```python
from build123d import *

# Parameters (mm, degrees)
SKETCH20_W            = 96.52
SKETCH20_H            = 108.5559932
BOSS_EXTRUDE5_DEPTH   = 1.699999902
BOSS_EXTRUDE6_DEPTH   = 1.7
FILLET3_R             = 2.54
F_4_40_TAPPED_HOLE3_D = 2.2606
SKETCH28_W            = 11.938
SKETCH28_H            = 11.938
SKETCH28_W_2          = 5.08
SKETCH28_H_2          = 5.08
SKETCH28_W_3          = 51.308
SKETCH28_H_3          = 77.978
SKETCH28_R            = 1.27
CUT_EXTRUDE1_DEPTH    = 8.89


with BuildPart() as part:
    # Sketch20 → Boss-Extrude5 (new body)
    with BuildSketch(Plane(origin=(0, 0, 0), x_dir=(1, 0, 0), z_dir=(0, 1, 0))):
        with Locations((46.26, 74.0579966)):
            Rectangle(SKETCH20_W, SKETCH20_H)
    extrude(amount=-BOSS_EXTRUDE5_DEPTH)

    # Sketch20_3 → Boss-Extrude6 (add)
    with BuildSketch(Plane(origin=(0, 0, 0), x_dir=(1, 0, 0), z_dir=(0, 1, 0))):
        with BuildLine():
            Line((2.572, 21.812), (89.948, 21.812))
            ThreePointArc((89.948, 21.812), (90.691948776, 23.608051224), (92.488, 24.352))
            Line((92.488, 24.352), (92.488, 123.7639932))
            ThreePointArc((92.488, 123.7639932), (90.691948776, 124.507941976), (89.948, 126.3039932))
            Line((89.948, 126.3039932), (2.572, 126.3039932))
            ThreePointArc((2.572, 126.3039932), (1.828051224, 124.507941976), (0.032, 123.7639932))
            Line((0.032, 123.7639932), (0.032, 24.352))
            ThreePointArc((0.032, 24.352), (1.828051224, 23.608051224), (2.572, 21.812))
        make_face()
        with BuildLine():
            Line((3.624102448, 23.082), (88.895897552, 23.082))
            ThreePointArc((88.895897552, 23.082), (89.793923164, 24.506076836), (91.218, 25.404102448))
            Line((91.218, 25.404102448), (91.218, 122.711890752))
            ThreePointArc((91.218, 122.711890752), (89.793923164, 123.609916364), (88.895897552, 125.0339932))
            Line((88.895897552, 125.0339932), (3.624102448, 125.0339932))
            ThreePointArc((3.624102448, 125.0339932), (2.726076836, 123.609916364), (1.302, 122.711890752))
            Line((1.302, 122.711890752), (1.302, 25.404102448))
            ThreePointArc((1.302, 25.404102448), (2.726076836, 24.506076836), (3.624102448, 23.082))
        make_face(mode=Mode.SUBTRACT)
    extrude(amount=BOSS_EXTRUDE6_DEPTH)

    # Fillet3
    fillet3_edges = [part.edges().sort_by_distance(p)[0] for p in [
        (-2, -0.849999951, -128.3359932),
        (-2, -0.849999951, -19.78),
        (94.52, -0.849999951, -19.78),
        (94.52, -0.849999951, -128.3359932),
    ]]
    fillet(fillet3_edges, radius=FILLET3_R)

    # 4-40 Tapped Hole3 (through all)
    with Locations(Plane(origin=(0, 0, 0), x_dir=(1, 0, 0), z_dir=(0, 1, 0))):
        with Locations((0.032, 21.812), (92.488, 21.812), (92.488, 126.3039932), (0.032, 126.3039932)):
            Hole(F_4_40_TAPPED_HOLE3_D / 2)

    # Sketch28 → Cut-Extrude1 (cut)
    with BuildSketch(Plane.XZ.offset(1.699999902)):
        with Locations((11.843, -110.331)):
            Rectangle(SKETCH28_W, SKETCH28_H)
        with Locations((10.954, -77.692)):
            Rectangle(SKETCH28_W_2, SKETCH28_H_2)
        with Locations((55.658, -74.009)):
            Rectangle(SKETCH28_W_3, SKETCH28_H_3)
        with Locations((87.662, -118.078)):
            Circle(SKETCH28_R)
        with Locations((87.662, -29.94)):
            Circle(SKETCH28_R)
        with Locations((23.019, -118.078)):
            Circle(SKETCH28_R)
        with Locations((23.019, -29.94)):
            Circle(SKETCH28_R)
    extrude(amount=-CUT_EXTRUDE1_DEPTH, mode=Mode.SUBTRACT)


solid = part.part
```
Model file for the job. Use its own axes, mm. A direction names the side the tool comes from. Round coordinates to 2 decimals unless told otherwise and drop trailing zeros. Loops run counter-clockwise (first coordinate to the right, second up) from the corner with the lowest first, then second, coordinate; pieces in that order, holes last. Notation, with made-up numbers: M 75,47.25 L 118,47.25 A18 ccw 118,72.25 Z; hole C 49.5,87 d4. An arc over 180 degrees is marked long. Put each result on its own line as item: value. Start each with the question number.
Item 1: Cut at C-C (z = -29.94). List the corners of the cut face in (x, y).
Item 2: Cut at A-A (z = -114.5). List the corners of the cut face in (x, y), then the cut area to 3 significant figures.
Item 3: Drill centre lines: line 1 along X through (y, z) = (-0.85, -106); line 2 along X through (y, z) = (0.9, -94.5); line 3 along Z through (x, y) = (38.5, 0.85). Where is each one in solid material? Low to high.
Item 4: Drop flat-ended pins along their axis: P1, Ø0.5, axis at x = 34, y = 0.5, coming from the -Z side; P2, Ø4, axis at x = 23.019, z = -29.94, coming from the -Y side; P3, Ø5, axis at x = 61.5, z = -31, coming from the +Y side; P4, Ø1.4, axis at y = 1, z = -93.5, coming from the -X side. Give the stop position or say it passes through.
Item 5: 3-axis set-ups, long thin cutter, end or side, ignore diameter. For faces 4 (the face through (93.756, -0.862, -20.504)), 5 (the face through (1.808, 0.838, -23.628)), 6 (the face through (2.743, 0.838, -123.627)): which of +Z, -Z, +X, -X, +Y, -Y reach the whole face in a straight line?
Item 6: Cut at B-B (x = 32). List the corners of the cut face in (y, z).
Item 7: Mould opens along Z. For faces 1 (the face through (26, 0, -75)), 2 (the face through (1.85, 0.84, -124.53)), 3 (the face through (46, 0, -127)) say: released by +Z, released by -Z, zero draft, split by the parting line, or undercut.
Item 8: Cut at D-D (y = 0.55). List the corners of the cut face in (x, z).
Answer block:
1. outline: M -2,-1.7 L 21.75,-1.7 L 21.75,0 L 1.3,0 L 1.3,1.7 L 0.03,1.7 L 0.03,0 L -2,0 Z; M 24.29,-1.7 L 86.39,-1.7 L 86.39,0 L 24.29,0 Z; M 88.93,-1.7 L 94.52,-1.7 L 94.52,0 L 92.49,0 L 92.49,1.7 L 91.22,1.7 L 91.22,0 L 88.93,0 Z
2. outline: M -2,-1.7 L 5.87,-1.7 L 5.87,0 L 1.3,0 L 1.3,1.7 L 0.03,1.7 L 0.03,0 L -2,0 Z; M 17.81,-1.7 L 94.52,-1.7 L 94.52,0 L 92.49,0 L 92.49,1.7 L 91.22,1.7 L 91.22,0 L 17.81,0 Z
2. area: 148 mm2
3. line 1: -2 to 5.87, 17.81 to 30, 81.31 to 94.52
3. line 2: 0.03 to 1.3, 91.22 to 92.49
3. line 3: -126.3 to -125.03, -23.08 to -21.81
4. P1: z = -126.3
4. P2: y = -1.7
4. P3: y = 0
4. P4: x = 0.03
5. face 4: +Z, +X, +Y, -Y
5. face 5: +Z, -X, +Y
5. face 6: +Y
6. outline: M -1.7,-128.34 L 0,-128.34 L 0,-126.3 L 1.7,-126.3 L 1.7,-125.03 L 0,-125.03 L 0,-113 L -1.7,-113 Z; M -1.7,-35.02 L 0,-35.02 L 0,-23.08 L 1.7,-23.08 L 1.7,-21.81 L 0,-21.81 L 0,-19.78 L -1.7,-19.78 Z
7. face 1: undercut
7. face 2: released by -Z
7. face 3: zero draft
8. outline: M 0.03,-123.76 A2.54 cw 2.57,-126.3 L 89.95,-126.3 A2.54 cw 92.49,-123.76 L 92.49,-24.35 A2.54 cw 89.95,-21.81 L 2.57,-21.81 A2.54 cw 0.03,-24.35 Z; hole M 1.3,-122.71 A3.81 cw 3.62,-125.03 L 88.9,-125.03 A3.81 cw 91.22,-122.71 L 91.22,-25.4 A3.81 cw 88.9,-23.08 L 3.62,-23.08 A3.81 cw 1.3,-25.4 Z
